```python
from build123d import *

# Parameters (mm, degrees)
SKETCH1_R           = 12.5
BOSS_EXTRUDE1_DEPTH = 18
SKETCH2_W           = 13
SKETCH2_H           = 15
CUT_EXTRUDE1_DEPTH  = 18
SKETCH3_R           = 2
SKETCH3_R_2         = 1
CUT_EXTRUDE2_DEPTH  = 26.228951623
BOSS_EXTRUDE2_DEPTH = 10


with BuildPart() as part:
    # Sketch1 → Boss-Extrude1 (new body)
    with BuildSketch(Plane(origin=(0, 0, 0), x_dir=(1, 0, 0), z_dir=(0, 1, 0))):
        with Locations(Location((0, 0, 0), (0, 0, 270))):
            Circle(SKETCH1_R)
    extrude(amount=BOSS_EXTRUDE1_DEPTH)

    # Sketch2 → Cut-Extrude1 (cut)
    with BuildSketch(Plane(origin=(0, 0, 0), x_dir=(0, 0, -1), z_dir=(1, 0, 0))):
        with Locations((0, 9)):
            Rectangle(SKETCH2_W, SKETCH2_H)
    extrude(amount=CUT_EXTRUDE1_DEPTH, mode=Mode.SUBTRACT)

    # Sketch3 → Cut-Extrude2 (cut, through all)
    # profile 1 of 2: a face of its own
    with BuildSketch(Plane.XZ):
        with Locations(Location((5, 0, 0), (0, 0, 270))):
            Circle(SKETCH3_R)
        with Locations((5, 0)):
            Circle(SKETCH3_R_2, mode=Mode.SUBTRACT)
    # profile 2 of 2: a face of its own
    with BuildSketch(Plane.XZ):
        with Locations((5, 0)):
            Circle(SKETCH3_R_2)
    extrude(amount=-CUT_EXTRUDE2_DEPTH, mode=Mode.SUBTRACT)

    # Sketch5 → Boss-Extrude2 (add)
    with BuildSketch(Plane.XZ):
        with BuildLine():
            Line((-1.414213562, 0.5), (-2.514213562, 0.5))
            Line((-2.514213562, 0.5), (-2.514213562, -0.5))
            Line((-2.514213562, -0.5), (-1.414213562, -0.5))
            ThreePointArc((-1.414213562, -0.5), (1.5, 0), (-1.414213562, 0.5))
        make_face()
    extrude(amount=BOSS_EXTRUDE2_DEPTH)


solid = part.part
```
Part model, mm, in its own coordinate system. A direction names the side the tool comes from. Round coordinates to 2 decimals unless told otherwise and drop trailing zeros. Write each loop counter-clockwise with the first axis right and the second up, starting at its lowest first coordinate (ties: lowest second). Pieces come first, ordered by that corner, then holes. Notation, with made-up numbers: M -39,36.25 L -17,36.25 A19 ccw -17,48.25 Z; hole C -12,16 d2. An arc over 180 degrees is marked long. Answer as CSV lines item,"result". Start each with the question number.
1) Which spindle directions (+Z, -Z, +X, -X, +Y, -Y) get a long thin tool onto all of the face, cutting with end or side? Do faces 1 (the face through (-2.514, -5, 0)), 2 (the face through (8, 16.5, 0)), 3 (the face through (1.5, -4.93, -0.06)), 4 (the face through (-2, -5, 0.5)), 5 (the face through (-2, -5, -0.5)). Say none if no direction does.
2) Band-saw the part on A-A (z = 0). List the corners of the cut face in (x, y).
3) Band-saw the part on C-C (y = -4). List the corners of the cut face in (x, z), then the cut area to 3 significant figures.
4) Band-saw the part on D-D (z = 4). List the corners of the cut face in (x, y).
5) Band-saw the part on B-B (x = 5). List the corners of the cut face in (y, z), then the cut area to 3 significant figures.
6) Mould opens along Y. For faces 6 (the face through (5, 9, -6.5)), 7 (the face through (5, 9, 6.5)), 8 (the face through (7, 1, 0)), 9 (the face through (0, 18, 0)) say: +Y half, -Y half, draft (parallel to the pull), parting line (faces both ways), or undercut.
7) Drill centre lines: L1, parallel to Y at x = 11.25, z = -4.75; L2, parallel to X at y = 0.75, z = 0; L3, parallel to Y at x = -1.5, z = 7.75. Where is each one in solid material? Low to high.
8) Drop flat-ended pins along their axis: pin 1 (0.9 mm diameter, centred on x = -2, y = -6, fed in from -Z); pin 2 (7.5 mm diameter, centred on x = -4, z = -5.5, fed in from -Y); pin 3 (4.5 mm diameter, centred on x = 5, z = 0, fed in from +Y); pin 4 (1.5 mm diameter, centred on y = 5, z = -8.5, fed in from +X). Give the stop position or say it passes through.
Worked out:
1,face 1,"+Z, -Z, -X, -Y"
1,face 2,"+X"
1,face 3,"-Y"
1,face 4,"+Z, -X, -Y"
1,face 5,"-Z, -X, -Y"
2,outline,"M -12.5,0 L -2.51,0 L -2.51,-10 L 1.5,-10 L 1.5,0 L 3,0 L 3,1.5 L 0,1.5 L 0,16.5 L 3,16.5 L 3,18 L -12.5,18 Z; M 7,0 L 12.5,0 L 12.5,1.5 L 7,1.5 Z; M 7,16.5 L 12.5,16.5 L 12.5,18 L 7,18 Z"
3,outline,"M -2.51,-0.5 L -1.41,-0.5 A1.5 ccw long -1.41,0.5 L -2.51,0.5 Z"
3,area,"8.11 mm²"
4,outline,"M -11.84,0 L 11.84,0 L 11.84,1.5 L 0,1.5 L 0,16.5 L 11.84,16.5 L 11.84,18 L -11.84,18 Z"
5,outline,"M 0,-11.46 L 18,-11.46 L 18,-2 L 16.5,-2 L 16.5,-6.5 L 1.5,-6.5 L 1.5,-2 L 0,-2 Z; M 0,2 L 1.5,2 L 1.5,6.5 L 16.5,6.5 L 16.5,2 L 18,2 L 18,11.46 L 0,11.46 Z"
5,area,"205 mm²"
6,face 6,"undercut"
6,face 7,"undercut"
6,face 8,"draft"
6,face 9,"+Y half"
7,L1,"0 to 1.5, 16.5 to 18"
7,L2,"-12.5 to 3, 7 to 12.5"
7,L3,"0 to 18"
8,pin 1,"z = -0.5"
8,pin 2,"y = 0"
8,pin 3,"y = 18"
8,pin 4,"x = 9.81"
